from build123d import *

# Parameters (mm, degrees)
ESQUISSE1_W             = 80
ESQUISSE1_H             = 170
BOSS_EXTRU_1_DEPTH      = 9
ESQUISSE2_R             = 1.25
ENL_V_MAT_EXTRU_1_DEPTH = 189.098378515
ESQUISSE4_W             = 28
ESQUISSE4_H             = 9
ENL_V_MAT_EXTRU_3_DEPTH = 189.098378515
ESQUISSE5_R             = 1.25
ENL_V_MAT_EXTRU_4_DEPTH = 10
ESQUISSE6_R             = 2.5
ENL_V_MAT_EXTRU_5_DEPTH = 189.098378515
CONG_1_R                = 4
ESQUISSE7_W             = 12
ESQUISSE7_H             = 9.1
ENL_V_MAT_EXTRU_6_DEPTH = 189.098378515
ESQUISSE8_R             = 1.6
ENL_V_MAT_EXTRU_7_DEPTH = 189.098378515


with BuildPart() as part:
    # Esquisse1 → Boss.-Extru.1 (new body)
    with BuildSketch(Plane.XY):
        with Locations((40, 85)):
            Rectangle(ESQUISSE1_W, ESQUISSE1_H)
    extrude(amount=BOSS_EXTRU_1_DEPTH)

    # Esquisse2 → Enlèv. mat.-Extru.1 (cut, through all)
    with BuildSketch(Plane.XY.offset(9)):
        with Locations((15, 10)):
            Circle(ESQUISSE2_R)
        with Locations(Location((65, 10, 0), (0, 0, 180))):
            Circle(ESQUISSE2_R)
        with Locations((15, 35)):
            Circle(ESQUISSE2_R)
        with Locations(Location((65, 35, 0), (0, 0, 180))):
            Circle(ESQUISSE2_R)
        with Locations((15, 60)):
            Circle(ESQUISSE2_R)
        with Locations(Location((65, 60, 0), (0, 0, 180))):
            Circle(ESQUISSE2_R)
        with Locations((15, 85)):
            Circle(ESQUISSE2_R)
        with Locations(Location((65, 85, 0), (0, 0, 180))):
            Circle(ESQUISSE2_R)
        with Locations((15, 110)):
            Circle(ESQUISSE2_R)
        with Locations(Location((65, 110, 0), (0, 0, 180))):
            Circle(ESQUISSE2_R)
        with Locations((15, 135)):
            Circle(ESQUISSE2_R)
        with Locations(Location((65, 135, 0), (0, 0, 180))):
            Circle(ESQUISSE2_R)
        with Locations((15, 160)):
            Circle(ESQUISSE2_R)
        with Locations(Location((65, 160, 0), (0, 0, 180))):
            Circle(ESQUISSE2_R)
        with Locations((15, 185)):
            Circle(ESQUISSE2_R)
        with Locations((65, 185)):
            Circle(ESQUISSE2_R)
    extrude(amount=-ENL_V_MAT_EXTRU_1_DEPTH, mode=Mode.SUBTRACT)

    # Esquisse4 → Enlèv. mat.-Extru.3 (cut, through all)
    with BuildSketch(Plane.XY.offset(9)):
        with Locations((40, 165.5)):
            Rectangle(ESQUISSE4_W, ESQUISSE4_H)
    extrude(amount=-ENL_V_MAT_EXTRU_3_DEPTH, mode=Mode.SUBTRACT)

    # Esquisse5 → Enlèv. mat.-Extru.4 (cut)
    with BuildSketch(Plane(origin=(0, 161, 0), x_dir=(1, 0, 0), z_dir=(0, 1, 0))):
        with Locations(Location((29, -4, 0), (0, 0, 270))):
            Circle(ESQUISSE5_R)
        with Locations(Location((51, -4, 0), (0, 0, 90))):
            Circle(ESQUISSE5_R)
    extrude(amount=-ENL_V_MAT_EXTRU_4_DEPTH, mode=Mode.SUBTRACT)

    # Esquisse6 → Enlèv. mat.-Extru.5 (cut, through all)
    with BuildSketch(Plane.XY.offset(9)):
        with Locations((74.8, 120.5)):
            Circle(ESQUISSE6_R)
        with Locations(Location((74.8, 60.5, 0), (0, 0, 180))):
            Circle(ESQUISSE6_R)
        with Locations((74.8, 100.5)):
            Circle(ESQUISSE6_R)
        with Locations(Location((74.8, 40.5, 0), (0, 0, 180))):
            Circle(ESQUISSE6_R)
        with Locations((5.2, 40.5)):
            Circle(ESQUISSE6_R)
        with Locations(Location((5.2, 100.5, 0), (0, 0, 180))):
            Circle(ESQUISSE6_R)
        with Locations((5.2, 60.5)):
            Circle(ESQUISSE6_R)
        with Locations(Location((5.2, 120.5, 0), (0, 0, 180))):
            Circle(ESQUISSE6_R)
        with Locations(Location((54.8, 100.5, 0), (0, 0, 180))):
            Circle(ESQUISSE6_R)
        with Locations(Location((54.8, 120.5, 0), (0, 0, 180))):
            Circle(ESQUISSE6_R)
        with Locations((54.8, 40.5)):
            Circle(ESQUISSE6_R)
        with Locations((54.8, 60.5)):
            Circle(ESQUISSE6_R)
        with Locations(Location((25.2, 60.5, 0), (0, 0, 180))):
            Circle(ESQUISSE6_R)
        with Locations(Location((25.2, 40.5, 0), (0, 0, 180))):
            Circle(ESQUISSE6_R)
        with Locations((25.2, 120.5)):
            Circle(ESQUISSE6_R)
        with Locations((25.2, 100.5)):
            Circle(ESQUISSE6_R)
    extrude(amount=-ENL_V_MAT_EXTRU_5_DEPTH, mode=Mode.SUBTRACT)

    # Congé1
    cong_1_edges = [part.edges().sort_by_distance(p)[0] for p in [
        (0, 170, 4.5),
        (80, 170, 4.5),
    ]]
    fillet(cong_1_edges, radius=CONG_1_R)

    # Esquisse7 → Enlèv. mat.-Extru.6 (cut, through all)
    with BuildSketch(Plane.XY.offset(9)):
        with Locations((16, 20.55)):
            Rectangle(ESQUISSE7_W, ESQUISSE7_H)
        with Locations((40, 20.55)):
            Rectangle(ESQUISSE7_W, ESQUISSE7_H)
        with Locations((64, 20.55)):
            Rectangle(ESQUISSE7_W, ESQUISSE7_H)
        with Locations((64, 92.65)):
            Rectangle(ESQUISSE7_W, ESQUISSE7_H)
        with Locations((40, 92.65)):
            Rectangle(ESQUISSE7_W, ESQUISSE7_H)
        with Locations((16, 92.65)):
            Rectangle(ESQUISSE7_W, ESQUISSE7_H)
    extrude(amount=-ENL_V_MAT_EXTRU_6_DEPTH, mode=Mode.SUBTRACT)

    # Esquisse8 → Enlèv. mat.-Extru.7 (cut, through all)
    with BuildSketch(Plane.XY.offset(9)):
        with Locations((11.080265456, 17.080265456)):
            Circle(ESQUISSE8_R)
        with Locations((11.080265456, 24.019734544)):
            Circle(ESQUISSE8_R)
        with Locations((20.919734544, 24.019734544)):
            Circle(ESQUISSE8_R)
        with Locations((20.919734544, 17.080265456)):
            Circle(ESQUISSE8_R)
        with Locations((35.080265456, 17.080265456)):
            Circle(ESQUISSE8_R)
        with Locations((35.080265456, 24.019734544)):
            Circle(ESQUISSE8_R)
        with Locations((44.919734544, 24.019734544)):
            Circle(ESQUISSE8_R)
        with Locations((44.919734544, 17.080265456)):
            Circle(ESQUISSE8_R)
        with Locations((59.080265456, 17.080265456)):
            Circle(ESQUISSE8_R)
        with Locations((59.080265456, 24.019734544)):
            Circle(ESQUISSE8_R)
        with Locations((68.919734544, 24.019734544)):
            Circle(ESQUISSE8_R)
        with Locations((68.919734544, 17.080265456)):
            Circle(ESQUISSE8_R)
        with Locations((68.919734544, 96.119734544)):
            Circle(ESQUISSE8_R)
        with Locations((68.919734544, 89.180265456)):
            Circle(ESQUISSE8_R)
        with Locations((59.080265456, 89.180265456)):
            Circle(ESQUISSE8_R)
        with Locations((59.080265456, 96.119734544)):
            Circle(ESQUISSE8_R)
        with Locations((44.919734544, 96.119734544)):
            Circle(ESQUISSE8_R)
        with Locations((44.919734544, 89.180265456)):
            Circle(ESQUISSE8_R)
        with Locations((35.080265456, 89.180265456)):
            Circle(ESQUISSE8_R)
        with Locations((35.080265456, 96.119734544)):
            Circle(ESQUISSE8_R)
        with Locations((20.919734544, 96.119734544)):
            Circle(ESQUISSE8_R)
        with Locations((20.919734544, 89.180265456)):
            Circle(ESQUISSE8_R)
        with Locations((11.080265456, 89.180265456)):
            Circle(ESQUISSE8_R)
        with Locations((11.080265456, 96.119734544)):
            Circle(ESQUISSE8_R)
        with Locations((27.080265456, 162.080265456)):
            Circle(ESQUISSE8_R)
        with Locations((52.919734544, 162.080265456)):
            Circle(ESQUISSE8_R)
    extrude(amount=-ENL_V_MAT_EXTRU_7_DEPTH, mode=Mode.SUBTRACT)


solid = part.part
Input: part model. Units: mm. Frame: model coordinates. Give positions to 0.01 mm unless a question says otherwise; leave off trailing zeros. Order: outer loops, then holes, each group sorted by start corner. A loop starts at its lowest first (then second) coordinate and runs counter-clockwise, first axis right, second up. Notation, with made-up numbers: M 27.5,-27.5 L 42.5,-27.5 A18 cw 42.5,-1.5 Z; hole C 81.25,7.25 d2. An arc over 180 degrees is marked long. Answer as a JSON object with one key per item and string values.
1. First-contact query: P1, Ø3, axis at x = 45, z = 2, coming from the +Y side; P2, Ø4, axis at x = 25.2, y = 100.5, coming from the +Z side. Flat tips, straight axial feed; report the tip coordinate or a pass-through.
Result sheet:
{"P1": "y = 161", "P2": "through"}
2. Cut plane A-A, the plane x = 39. Output: boundary loops of the cut face in (y, z), and give its area (3 significant figures).
Result sheet:
{"outline": "M 0,0 L 16,0 L 16,9 L 0,9 Z; M 25.1,0 L 88.1,0 L 88.1,9 L 25.1,9 Z; M 97.2,0 L 161,0 L 161,9 L 97.2,9 Z", "area": "1,290 mm²"}
3. Pull-direction query (Y, two-part tool) for faces 1 (the flat face through (16, 97.2, 5)), 2 (the flat face through (16, 16, 5)), 3 (the flat face through (15, 170, 4)); classes: +Y half, -Y half, draft (parallel to the pull), parting line (faces both ways), or undercut.
Result sheet:
{"face 1": "undercut", "face 2": "undercut", "face 3": "+Y half"}
4. Ray query, line 1 (Y direction, x = 5.2, z = 2); line 2 (Y direction, x = 37.5, z = 5.75); line 3 (X direction, y = 85, z = 5.5). Return the intervals inside material, ascending. Write a range as [from, to].
Result sheet:
{"line 1": "[0, 38], [43, 58], [63, 98], [103, 118], [123, 170]", "line 2": "[0, 16], [25.1, 88.1], [97.2, 161]", "line 3": "[0, 13.75], [16.25, 63.75], [66.25, 80]"}
5. Cut plane B-B, the plane y = 120.5. Output: boundary loops of the cut face in (x, z).
Result sheet:
{"outline": "M 0,0 L 2.7,0 L 2.7,9 L 0,9 Z; M 7.7,0 L 22.7,0 L 22.7,9 L 7.7,9 Z; M 27.7,0 L 52.3,0 L 52.3,9 L 27.7,9 Z; M 57.3,0 L 72.3,0 L 72.3,9 L 57.3,9 Z; M 77.3,0 L 80,0 L 80,9 L 77.3,9 Z"}
